Input: dimensioned drawing with shaded views. Units: mm. Origin: part minimum x, y, z. A direction names the side the tool comes from. Round coordinates to 2 decimals unless told otherwise and drop trailing zeros. Order: outer loops, then holes, each group sorted by start corner. A loop starts at its lowest first (then second) coordinate and runs counter-clockwise, first axis right, second up.
Item 1: Line query: L1, parallel to Z at x = 8, y = 13 (1 decimal); L2, parallel to Y at x = 24, z = 4.5; L3, parallel to X at y = 21, z = 6.5 (1 decimal). Output: solid intervals per line, ascending.
Item 2: First-contact query: pin 1 (2 mm diameter, centred on x = 21.5, z = 66, fed in from +Y); pin 2 (1.5 mm diameter, centred on y = 19, z = 64.5, fed in from +X); pin 3 (6 mm diameter, centred on y = 26, z = 44.5, fed in from +X). Flat tips, straight axial feed; report the tip coordinate or a pass-through.
Item 3: Cut plane A-A on y = 32. Output: boundary loops of the cut face in (x, z) (1 decimal), then the cut area to 3 significant figures.
Item 4: Cut plane C-C on z = 22. Output: boundary loops of the cut face in (x, y).
Item 5: Reachability of the marked faces 1 and 2 from +Z, -Z, +X, -X, +Y, -Y: full face, straight path, thin tool, end or side. Return the list, or none.
Item 6: Cut plane D-D on x = 6. Output: boundary loops of the cut face in (y, z) (1 decimal).
Item 7: Cut plane B-B on x = 18.5. Output: boundary loops of the cut face in (y, z) (1 decimal).
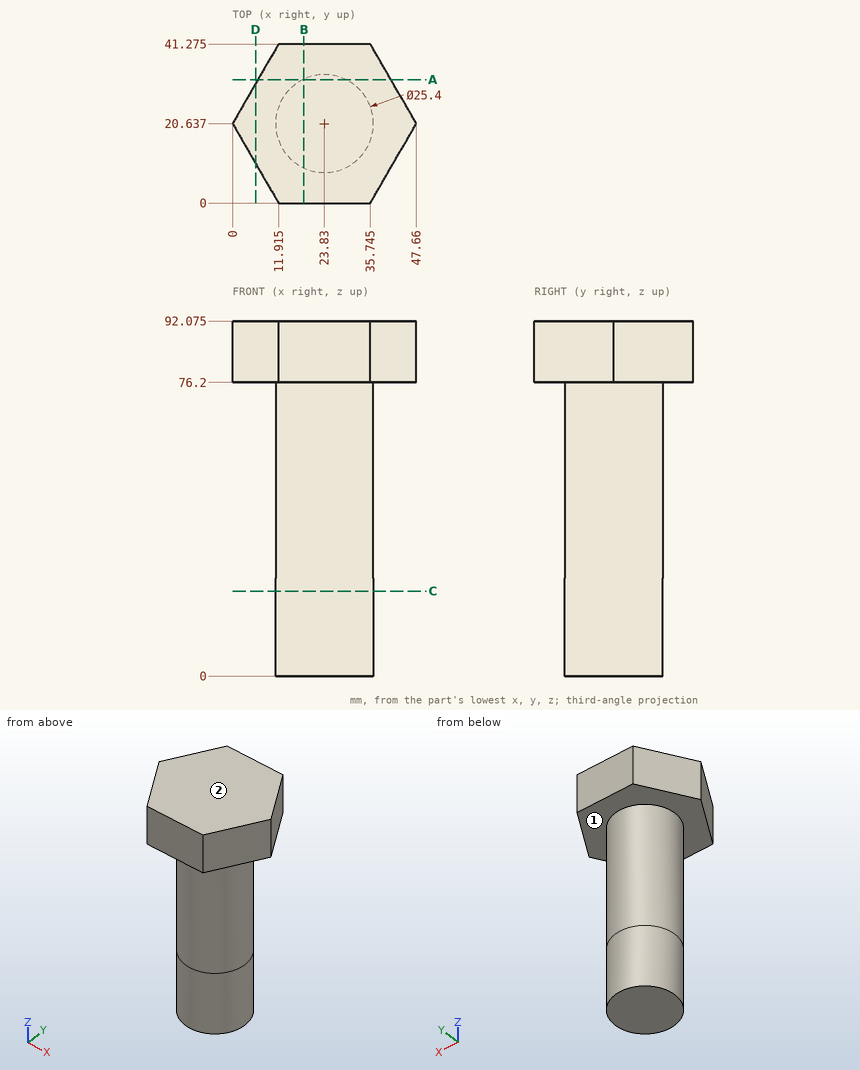
From the geometry:
1. L1: z = 76.2 to 92.1
1. L2: y = 7.94 to 33.34
1. L3: x = 11.1 to 36.5
2. pin 1: stops at y = 33.27
2. pin 2: stops at x = 36.5
2. pin 3: stops at x = 36.31
3. outline: (6.6, 76.2) - (18.2, 76.2) - (18.2, 0) - (29.5, 0) - (29.5, 76.2) - (41.1, 76.2) - (41.1, 92.1) - (6.6, 92.1) - close
3. area: 1,410 mm2
4. outline: circle Ø25.4 at (23.83, 20.64)
5. face 1: -Z
5. face 2: +Z, +X, -X, +Y, -Y
6. outline: (10.2, 76.2) - (31, 76.2) - (31, 92.1) - (10.2, 92.1) - close
7. outline: (0, 76.2) - (9.1, 76.2) - (9.1, 0) - (32.2, 0) - (32.2, 76.2) - (41.3, 76.2) - (41.3, 92.1) - (0, 92.1) - close
